Design review of the part built by this model. Coordinates are the model's own, in mm. Face numbers are marked on the shaded views. Give positions to 0.01 mm unless a question says otherwise; leave off trailing zeros. Loops run counter-clockwise (first coordinate to the right, second up) from the corner with the lowest first, then second, coordinate; pieces in that order, holes last. Notation, with made-up numbers: M 32,8 L 58,8 A15 ccw 58,14 Z; hole C 73,7 d9. An arc over 180 degrees is marked long. Use one line per item in the form item = value. Start each with the question number.
from build123d import *

# Parameters (mm, degrees)
SKETCH1_W           = 50
SKETCH1_H           = 40
BOSS_EXTRUDE1_DEPTH = 10
SKETCH2_R           = 2.05
CUT_EXTRUDE1_DEPTH  = 10
SKETCH4_R           = 3.05
CUT_EXTRUDE2_DEPTH  = 10
SKETCH5_R           = 2
CUT_EXTRUDE3_DEPTH  = 10
SKETCH6_R           = 3.5
CUT_EXTRUDE4_DEPTH  = 4
SKETCH7_R           = 3.5
CUT_EXTRUDE5_DEPTH  = 4


with BuildPart() as part:
    # Sketch1 → Boss-Extrude1 (new body)
    with BuildSketch(Plane(origin=(0, 0, 0), x_dir=(1, 0, 0), z_dir=(0, 1, 0))):
        Rectangle(SKETCH1_W, SKETCH1_H)
    extrude(amount=BOSS_EXTRUDE1_DEPTH)

    # Sketch2 → Cut-Extrude1 (cut)
    with BuildSketch(Plane(origin=(0, 10, 0), x_dir=(1, 0, 0), z_dir=(0, 1, 0))):
        with Locations((20, 10)):
            Circle(SKETCH2_R)
    extrude(amount=-CUT_EXTRUDE1_DEPTH, mode=Mode.SUBTRACT)

    # Sketch4 → Cut-Extrude2 (cut)
    with BuildSketch(Plane(origin=(0, 10, 0), x_dir=(1, 0, 0), z_dir=(0, 1, 0))):
        with Locations((-15, 15)):
            Circle(SKETCH4_R)
        with Locations((5, 15)):
            Circle(SKETCH4_R)
    extrude(amount=-CUT_EXTRUDE2_DEPTH, mode=Mode.SUBTRACT)

    # Sketch5 → Cut-Extrude3 (cut)
    with BuildSketch(Plane(origin=(0, 10, 0), x_dir=(1, 0, 0), z_dir=(0, 1, 0))):
        with Locations((20, -15)):
            Circle(SKETCH5_R)
    extrude(amount=-CUT_EXTRUDE3_DEPTH, mode=Mode.SUBTRACT)

    # Sketch6 → Cut-Extrude4 (cut)
    with BuildSketch(Plane(origin=(0, 10, 0), x_dir=(1, 0, 0), z_dir=(0, 1, 0))):
        with Locations((20, 10)):
            Circle(SKETCH6_R)
    extrude(amount=-CUT_EXTRUDE4_DEPTH, mode=Mode.SUBTRACT)

    # Sketch7 → Cut-Extrude5 (cut)
    with BuildSketch(Plane(origin=(0, 10, 0), x_dir=(1, 0, 0), z_dir=(0, 1, 0))):
        with Locations((20, -15)):
            Circle(SKETCH7_R)
    extrude(amount=-CUT_EXTRUDE5_DEPTH, mode=Mode.SUBTRACT)


solid = part.part
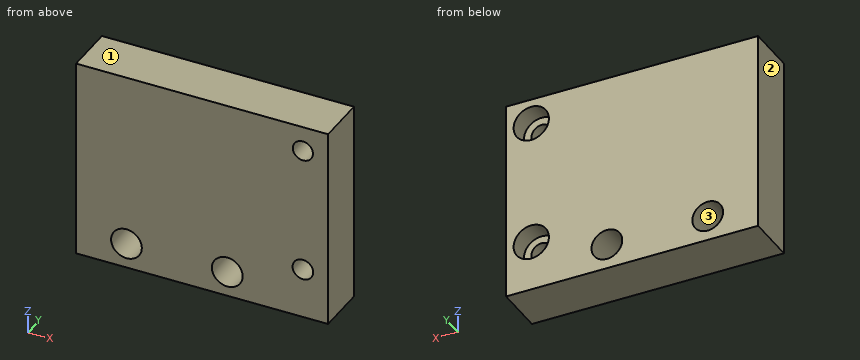
Q1. Take a section at B-B on x = 20. Give the boundary of the cut face in (y, z), plus the area to 3 significant figures.
Q2. Take a section at A-A on z = -15. Give the boundary of the cut face in (x, y), plus the area to 3 significant figures.
Q3. Take a section at D-D on x = 5. Give the boundary of the cut face in (y, z), plus the area to 3 significant figures.
Q4. Take a section at C-C on z = -10. Give the boundary of the cut face in (x, y).
Q5. Wall thickness on probe 1 along X at (y, z) = (5.25, -15); probe 2 along Z at (x, y) = (20, 8.55); probe 3 along Z at (x, y) = (20, 3.15): over which ranges is each line inside the solid? List them lowest first.
Q6. The part is to be moulded in two halves that separate along Z. For the marked faces 1, 2 and 3, say which applies: pulls with the +Z half, pulls with the -Z half, needs draft (parallel to the pull), parting line crosses it, or undercut.
Response values:
q1.outline = M 0,-20 L 10,-20 L 10,-13.5 L 6,-13.5 L 6,-12.05 L 0,-12.05 Z; M 0,-7.95 L 6,-7.95 L 6,-6.5 L 10,-6.5 L 10,11.5 L 6,11.5 L 6,13 L 0,13 Z; M 0,17 L 6,17 L 6,18.5 L 10,18.5 L 10,20 L 0,20 Z
q1.area = 295 mm^2
q2.outline = M -25,0 L -18.05,0 L -18.05,10 L -25,10 Z; M -11.95,0 L 1.95,0 L 1.95,10 L -11.95,10 Z; M 8.05,0 L 25,0 L 25,10 L 8.05,10 Z
q2.area = 378 mm^2
q3.outline = M 0,-20 L 10,-20 L 10,-18.05 L 0,-18.05 Z; M 0,-11.95 L 10,-11.95 L 10,20 L 0,20 Z
q3.area = 339 mm^2
q4.outline = M -25,0 L 17.95,0 L 17.95,6 L 16.5,6 L 16.5,10 L -25,10 Z; M 22.05,0 L 25,0 L 25,10 L 23.5,10 L 23.5,6 L 22.05,6 Z
q5.probe_1 = -25 to -18.05, -11.95 to 1.95, 8.05 to 25
q5.probe_2 = -20 to -13.5, -6.5 to 11.5, 18.5 to 20
q5.probe_3 = -20 to -12.05, -7.95 to 13, 17 to 20
q6.face_1 = pulls with the +Z half
q6.face_2 = needs draft
q6.face_3 = undercut
